```python
from build123d import *

# Parameters (mm, degrees)
SKETCH1_W              = 90
SKETCH1_H              = 25
BOSS_EXTRUDE1_DEPTH    = 80
SKETCH_1_R             = 25
CUT_EXTRUDE_1_DEPTH    = 10.5
SKETCH_2_R             = 5
CUT_EXTRUDE_2_DEPTH    = 100
SKETCH_3_R             = 8
CUT_EXTRUDE_3_DEPTH    = 100
SKETCH_4_R             = 10
CUT_EXTRUDE_4_DEPTH    = 10.5
SKETCH_5_R             = 2.25
CUT_EXTRUDE_5_DEPTH    = 10.5
PATTERN_LINEAR_1_COUNT = 2
PATTERN_LINEAR_1_PITCH = 24


with BuildPart() as part:
    # Sketch1 → Boss-Extrude1 (new body)
    with BuildSketch(Plane.XY):
        with Locations((-0.130315501, 10.641289438)):
            Rectangle(SKETCH1_W, SKETCH1_H)
    extrude(amount=BOSS_EXTRUDE1_DEPTH)

    # Эскиз1 → Вырез-Вытянуть1 (cut)
    with BuildSketch(Plane.XZ.offset(1.858710562)):
        with Locations(Location((-5.130315501, 33, 0), (0, 0, 270))):
            Circle(SKETCH_1_R)
    extrude(amount=-CUT_EXTRUDE_1_DEPTH, mode=Mode.SUBTRACT)

    # Эскиз2 → Вырез-Вытянуть2 (cut)
    with BuildSketch(Plane.XZ.offset(-8.641289438)):
        with Locations(Location((-5.130315501, 33, 0), (0, 0, 270))):
            Circle(SKETCH_2_R)
    extrude(amount=-CUT_EXTRUDE_2_DEPTH, mode=Mode.SUBTRACT)

    # Эскиз3 → Вырез-Вытянуть3 (cut)
    with BuildSketch(Plane.XZ.offset(1.858710562)):
        with Locations(Location((-25.130315501, 52, 0), (0, 0, 270))):
            Circle(SKETCH_3_R)
    extrude(amount=-CUT_EXTRUDE_3_DEPTH, mode=Mode.SUBTRACT)

    # Эскиз4 → Вырез-Вытянуть4 (cut)
    with BuildSketch(Plane.XZ.offset(1.858710562)):
        with Locations((-25.130315501, 52)):
            Circle(SKETCH_4_R)
    extrude(amount=-CUT_EXTRUDE_4_DEPTH, mode=Mode.SUBTRACT)

    # Эскиз5 → Вырез-Вытянуть5 (cut)
    with BuildSketch(Plane(origin=(0, 23.141289438, 0), x_dir=(1, 0, 0), z_dir=(0, 1, 0))):
        with Locations(Location((-37.130315501, -52, 0), (0, 0, 270))):
            Circle(SKETCH_5_R)
    cut_extrude_5 = extrude(amount=-CUT_EXTRUDE_5_DEPTH, mode=Mode.SUBTRACT)

    # Линейный массив1: Вырез-Вытянуть5 ×2
    with Locations(*[(i * PATTERN_LINEAR_1_PITCH, 0, 0) for i in range(1, PATTERN_LINEAR_1_COUNT)]):
        add(cut_extrude_5, mode=Mode.SUBTRACT)


solid = part.part
```
Model file for the job. Use its own axes, mm. A direction names the side the tool comes from. Coordinates: 2 decimals unless noted, no trailing zeros. Loops run counter-clockwise (first coordinate to the right, second up) from the corner with the lowest first, then second, coordinate; pieces in that order, holes last. Notation, with made-up numbers: (61, 13) - (65, 13) arc R13 ccw to (65, 28) - close; hole circle Ø8 at (84, -28). An arc over 180 degrees is marked (long way). Answer as a JSON object with one key per item and string values. Group by question number.
(1) Tool access for faces 1 (the face through (-37, 12.641, 52)), 2 (the face through (-32.94, 15.79, 53.73)), 3 (the face through (-1, 8.641, 29)): list every direction of +Z, -Z, +X, -X, +Y, -Y with a clear straight run to the whole face (end or side of a thin tool).
(2) Probe line 1 along X through (y, z) = (15.25, 52); line 2 along X through (y, z) = (12.75, 33); line 3 along X through (y, z) = (1, 33). List the from-to ranges inside material, lowest first.
(3) Cut at C-C (y = 19.25). Give the cut face in (x, z).
(4) Flat gauge pins, fed straight in: pin 1 (3.5 mm diameter, centred on x = -13, z = 52, fed in from +Y); pin 2 (18.5 mm diameter, centred on x = -25.13, z = 52, fed in from -Y); pin 3 (8 mm diameter, centred on x = -5.13, z = 33, fed in from +Y). Where does each tip first touch, or does it go through?
(5) Cut at A-A (z = 33). Give the cut face in (x, y), then the cut area to 3 significant figures.
(6) Cut at B-B (x = -3.5). Give the cut face in (y, z).
(7) Cut at D-D (x = 12). Give the cut face in (y, z), then the cut area to 3 significant figures.
(8) Two-plate mould, pull along X, no slides. Class faces 4 (the face through (-45.13, 10, 39)), 5 (the face through (-1, 11, 0)), 6 (the face through (-13.031, 17.965, 49.752)): released by +X, released by -X, zero draft, split by the parting line, or undercut.
Geometry says:
{
 "1": {"face 1": "+Y", "face 2": "+Y, -Y", "face 3": "-Y"},
 "2": {"line 1": "x = -45.13 to -39.38, -34.88 to -33.13, -17.13 to -15.38, -10.88 to 44.87", "line 2": "x = -45.13 to -10.13, -0.13 to 44.87", "line 3": "x = -45.13 to -30.13, 19.87 to 44.87"},
 "3": {"outline": "(-45.13, 0) - (44.87, 0) - (44.87, 80) - (-45.13, 80) - close; hole circle Ø4.5 at (-37.13, 52); hole circle Ø16 at (-25.13, 52); hole circle Ø4.5 at (-13.13, 52); hole circle Ø10 at (-5.13, 33)"},
 "4": {"pin 1": "stops at y = 12.64", "pin 2": "stops at y = 8.64", "pin 3": "passes through"},
 "5": {"outline": "(-45.13, -1.86) - (-30.13, -1.86) - (-30.13, 8.64) - (-10.13, 8.64) - (-10.13, 23.14) - (-45.13, 23.14) - close; (-0.13, 8.64) - (19.87, 8.64) - (19.87, -1.86) - (44.87, -1.86) - (44.87, 23.14) - (-0.13, 23.14) - close", "area": "1,580 mm^2"},
 "6": {"outline": "(-1.86, 0) - (23.14, 0) - (23.14, 28.27) - (8.64, 28.27) - (8.64, 8.05) - (-1.86, 8.05) - close; (-1.86, 57.95) - (8.64, 57.95) - (8.64, 37.73) - (23.14, 37.73) - (23.14, 80) - (-1.86, 80) - close"},
 "7": {"outline": "(-1.86, 0) - (23.14, 0) - (23.14, 80) - (-1.86, 80) - (-1.86, 51.21) - (8.64, 51.21) - (8.64, 14.79) - (-1.86, 14.79) - close", "area": "1,620 mm^2"},
 "8": {"face 4": "released by -X", "face 5": "zero draft", "face 6": "undercut"}
}
